Check sheet for the modelled part. Datum: model origin and axes. Units: mm. A direction names the side the tool comes from. Round coordinates to 2 decimals unless told otherwise and drop trailing zeros. Loops run counter-clockwise (first coordinate to the right, second up) from the corner with the lowest first, then second, coordinate; pieces in that order, holes last. Notation, with made-up numbers: (-26.5, -13) -> (-4.5, -13) arc R30 cw to (-4.5, 13) -> close; hole circle Ø8 at (80, -19). An arc over 180 degrees is marked (long way). One line per question, with ' | ' between items.
```python
from build123d import *

# Parameters (mm, degrees)
SKETCH014_W        = 116.03
SKETCH014_H        = 64.17
SKETCH014_W_2      = 97.158283
SKETCH014_H_2      = 39.832356
EXTRUDE002_DEPTH   = 17
POCKET005004_DEPTH = 15
FILLET_R           = 9
SKETCH018_W        = 11
SKETCH018_H        = 2.6
POCKET005005_DEPTH = 5


with BuildPart() as part:
    # Sketch014 → Extrude002 (new body)
    with BuildSketch(Plane.XY):
        with Locations((5.870297, 0.068238)):
            Rectangle(SKETCH014_W, SKETCH014_H)
        with Locations((-0.027307, -0.001692)):
            Rectangle(SKETCH014_W_2, SKETCH014_H_2, mode=Mode.SUBTRACT)
    extrude(amount=EXTRUDE002_DEPTH)

    # Sketch017 (on Face10 of Extrude002) → Pocket005004 (cut)
    with BuildSketch(Plane.XY.offset(17)):
        with BuildLine():
            Line((-41.973666, 30.903742), (53.475128, 30.903742))
            ThreePointArc((62.221588, 22.157282), (59.659809, 28.341963), (53.475128, 30.903742))
            Line((62.221588, 22.157282), (62.221588, -23.433549))
            ThreePointArc((54.711295, -30.943842), (60.021874, -28.744128), (62.221588, -23.433549))
            Line((54.711295, -30.943842), (-43.311095, -30.943842))
            Line((-43.311095, -30.943842), (-50.860429, -30.943842))
            Line((-50.860429, -30.943842), (-50.860429, -23.394508))
            Line((-50.860429, -23.394508), (-50.860429, 22.016979))
            Line((-50.860429, 30.903742), (-50.860429, 22.016979))
            Line((-41.973666, 30.903742), (-50.860429, 30.903742))
        make_face()
    extrude(amount=-POCKET005004_DEPTH, mode=Mode.SUBTRACT)

    # Fillet
    fillet_edges = [part.edges().sort_by_distance(p)[0] for p in [
        (63.885297, 32.153238, 8.5),
        (63.885297, -32.016762, 8.5),
    ]]
    fillet(fillet_edges, radius=FILLET_R)

    # Sketch018 (on Face6 of Fillet) → Pocket005005 (cut)
    with BuildSketch(Plane.YZ.offset(63.885297)):
        with Locations((16.617887, 10.937535)):
            Rectangle(SKETCH018_W, SKETCH018_H)
    extrude(amount=-POCKET005005_DEPTH, mode=Mode.SUBTRACT)


solid = part.part
```
(1) Scan lines: probe 1 along Y at (x, z) = (8, 13.25); probe 2 along X at (y, z) = (-7, 15.5); probe 3 along Y at (x, z) = (14, 1.5). Record each from-to range of solid material in increasing order.
Answer:
probe 1: y = -32.02 to -30.94, 30.9 to 32.15 | probe 2: x = -52.14 to -50.86, 62.22 to 63.89 | probe 3: y = -32.02 to -19.92, 19.91 to 32.15
(2) Sectioned sample at C-C, the plane y = -10. Record the cut outline in (x, z).
Answer:
outline: (-52.14, 0) -> (-48.61, 0) -> (-48.61, 2) -> (-50.86, 2) -> (-50.86, 17) -> (-52.14, 17) -> close; (48.55, 0) -> (63.89, 0) -> (63.89, 17) -> (62.22, 17) -> (62.22, 2) -> (48.55, 2) -> close
(3) Sectioned sample at B-B, the plane y = 14. Record the cut outline in (x, z), and give its area (3 significant figures).
Answer:
outline: (-52.14, 0) -> (-48.61, 0) -> (-48.61, 2) -> (-50.86, 2) -> (-50.86, 17) -> (-52.14, 17) -> close; (48.55, 0) -> (63.89, 0) -> (63.89, 9.64) -> (62.22, 9.64) -> (62.22, 2) -> (48.55, 2) -> close; (62.22, 12.24) -> (63.89, 12.24) -> (63.89, 17) -> (62.22, 17) -> close | area: 77.6 mm2
(4) Go/stop test with flat-tipped pins: pin 1 (1.8 mm diameter, centred on x = 63, z = 11.5, fed in from +Y); pin 2 (0.5 mm diameter, centred on x = 63, z = 11, fed in from -Y); pin 3 (8 mm diameter, centred on x = -21, y = -14, fed in from -Z); pin 4 (8 mm diameter, centred on x = -22, y = -17, fed in from +Z). Record where each tip stops, or that it passes through.
Answer:
pin 1: stops at y = 28.53 | pin 2: stops at y = -27.39 | pin 3: passes through | pin 4: stops at z = 2
(5) Sectioned sample at D-D, the plane z = 8.5. Record the cut outline in (x, y), and give its area (3 significant figures).
Answer:
outline: (-52.14, -32.02) -> (54.89, -32.02) arc R9 ccw to (63.89, -23.02) -> (63.89, 23.15) arc R9 ccw to (54.89, 32.15) -> (-52.14, 32.15) -> close; hole (-50.86, -30.94) -> (54.71, -30.94) arc R7.51 ccw to (62.22, -23.43) -> (62.22, 22.16) arc R8.75 ccw to (53.48, 30.9) -> (-50.86, 30.9) -> close | area: 446 mm2
(6) Mould release check, pull along Y, two halves, no side actions. Record for faces 3 (the face through (1, -32.017, 8)), 4 (the face through (5, 22, 0)), 5 (the face through (2, 30.904, 10)): +Y half, -Y half, draft (parallel to the pull), parting line (faces both ways), or undercut.
Answer:
face 3: -Y half | face 4: draft | face 5: undercut
(7) Set-up check for faces 1 (the face through (62.222, 0, 10)), 2 (the face through (-52.145, 0, 8)): record each of +Z, -Z, +X, -X, +Y, -Y from which the full face is reachable in a straight line by a thin tool's end or side.
Answer:
face 1: +Z | face 2: +Z, -Z, -X, +Y, -Y
(8) Sectioned sample at A-A, the plane x = -37. Record the cut outline in (y, z), and give its area (3 significant figures).
Answer:
outline: (-32.02, 0) -> (-19.92, 0) -> (-19.92, 2) -> (-30.94, 2) -> (-30.94, 17) -> (-32.02, 17) -> close; (19.91, 0) -> (32.15, 0) -> (32.15, 17) -> (30.9, 17) -> (30.9, 2) -> (19.91, 2) -> close | area: 83.5 mm2
